```python
from build123d import *

# Parameters (mm, degrees)
F0_W     = 41
F0_H     = 12
F0_R     = 1.5
F0_W_2   = 5
F1_DEPTH = 2.1
F2_DEPTH = 25
F3_R     = 2
F4_DEPTH = 12.5
F5_R     = 5.99999
F6_R     = 8


# Not quite as in the source:
# - a fillet or chamfer is up to 0.001 mm smaller than in the source, because OpenCascade refuses the exact size


with BuildPart() as f1:
    # F0 (on Top) → F1 (new body)
    with BuildSketch(Plane.XY):
        with Locations((-23, 0)):
            Rectangle(F0_W, F0_H)
        with Locations((-39, 0)):
            Circle(F0_R, mode=Mode.SUBTRACT)
        Rectangle(F0_W_2, F0_H)
        with Locations((23, 0)):
            Rectangle(F0_W, F0_H)
        with Locations((39, 0)):
            Circle(F0_R, mode=Mode.SUBTRACT)
    extrude(amount=F1_DEPTH)

    # F0 (on Top) → F2 (join)
    with BuildSketch(Plane.XY):
        Rectangle(F0_W_2, F0_H)
    extrude(amount=F2_DEPTH)

    # F3 (on Right) → F4 (cut, symmetric)
    with BuildSketch(Plane.YZ):
        with Locations((0, 18)):
            Circle(F3_R)
    extrude(amount=F4_DEPTH, both=True, mode=Mode.SUBTRACT)

    # F5 (radius 6 in the source; OpenCascade refuses exactly that, so slightly less here)
    f5_edges = [f1.edges().sort_by_distance(p)[0] for p in [
        (0, -6, 25),
        (0, 6, 25),
        (-43.5, -6, 1.05),
        (-43.5, 6, 1.05),
        (43.5, -6, 1.05),
        (43.5, 6, 1.05),
    ]]
    fillet(f5_edges, radius=F5_R)

    # F6
    f6_edges = [f1.edges().sort_by_distance(p)[0] for p in [
        (2.5, 0, 2.1),
        (-2.5, 0, 2.1),
    ]]
    fillet(f6_edges, radius=F6_R)


solid = f1.part
```
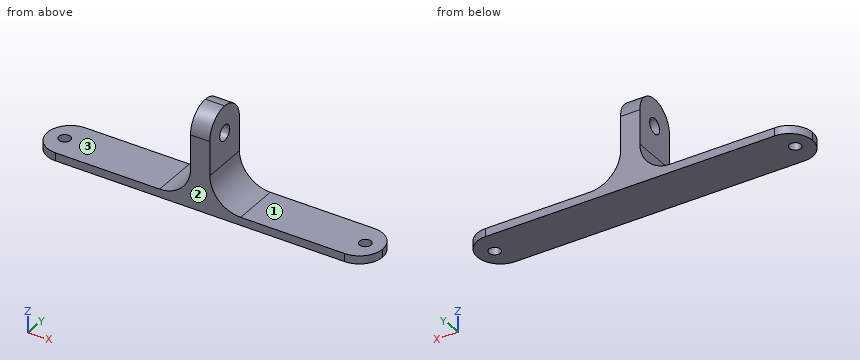
Part model, mm, in its own coordinate system. Face numbers are marked on the shaded views. A direction names the side the tool comes from. Give positions to 0.01 mm unless a question says otherwise; leave off trailing zeros. Order: outer loops, then holes, each group sorted by start corner. A loop starts at its lowest first (then second) coordinate and runs counter-clockwise, first axis right, second up. Notation, with made-up numbers: (45, 79.25) - (60, 79.25) arc R16 cw to (60, 109.25) - close; hole circle Ø1 at (-20.5, -14). An arc over 180 degrees is marked (long way). Use one line per item in the form item = value.
Item 1: Which spindle directions (+Z, -Z, +X, -X, +Y, -Y) get a long thin tool onto all of the face, cutting with end or side? Do the marked faces 1, 2 and 3. Say none if no direction does.
Solution:
face_1 = +Z, +X, +Y, -Y
face_2 = +Z, -Z, +X, -X, -Y
face_3 = +Z, -X, +Y, -Y
Item 2: Slice it at C-C on x = 39. Give the cut face in (y, z).
Solution:
outline = (-5.81, 0) - (-1.5, 0) - (-1.5, 2.1) - (-5.81, 2.1) - close; (1.5, 0) - (5.81, 0) - (5.81, 2.1) - (1.5, 2.1) - close
Item 3: Slice it at D-D on x = -16. Give the cut face in (y, z), and give its area (3 significant figures).
Solution:
outline = (-6, 0) - (6, 0) - (6, 2.1) - (-6, 2.1) - close
area = 25.2 mm2
Item 4: Pin check, flat tips, straight feed: pin 1 Ø1 at (x, y) = (-31.5, 3) entering from +Z; pin 2 Ø3.5 at (y, z) = (-1, 19.5) entering from +X; pin 3 Ø3.5 at (y, z) = (2, 15) entering from -X; pin 4 Ø2 at (y, z) = (0.5, 17.5) entering from -X. Stop position of each tip, or through.
Solution:
pin_1 = 2.1
pin_2 = 2.5
pin_3 = -2.5
pin_4 = through
Item 5: Probe probe 1 along Z at (x, y) = (-26, -4.5); probe 2 along Z at (x, y) = (-8, 1.5); probe 3 along X at (y, z) = (-0.5, 15.75). List the from-to ranges inside material, lowest first. Write a range as from..to.
Solution:
probe_1 = 0..2.1
probe_2 = 0..2.5
probe_3 = -2.5..2.5
Item 6: Slice it at A-A on z = 18. Give the cut face in (x, y).
Solution:
outline = (-2.5, -6) - (2.5, -6) - (2.5, -2) - (-2.5, -2) - close; (-2.5, 2) - (2.5, 2) - (2.5, 6) - (-2.5, 6) - close
